For this review, use the dimensioned drawing (mm, ordinates from the lowest corner) and the shaded views. A direction names the side the tool comes from. Round coordinates to 2 decimals unless told otherwise and drop trailing zeros. Write each loop counter-clockwise with the first axis right and the second up, starting at its lowest first coordinate (ties: lowest second). Pieces come first, ordered by that corner, then holes. Notation, with made-up numbers: M 39.25,-11.75 L 81.25,-11.75 A29 cw 81.25,18.25 Z; hole C 7,56.5 d11. An arc over 180 degrees is marked long. One line per question, with ' | ' between items.
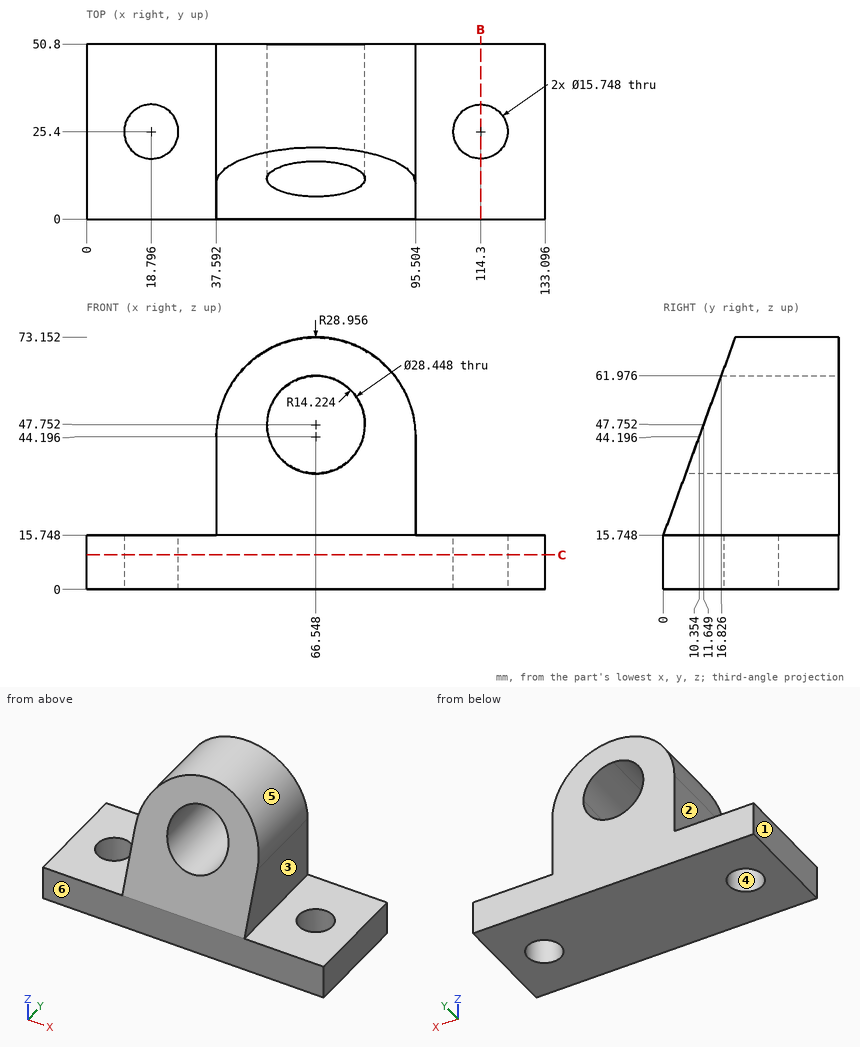
Item 1: Take a section at B-B (x = 114.3). Write out the cut boundary in (y, z) (1 decimal).
Results:
outline: M 0,0 L 17.5,0 L 17.5,15.7 L 0,15.7 Z; M 33.3,0 L 50.8,0 L 50.8,15.7 L 33.3,15.7 Z
Item 2: Machinability: for the marked faces 1, 2 and 3, which of the approach directions +Z, -Z, +X, -X, +Y, -Y give a long, thin tool a straight path to every point of the face, cutting with its end or side? Answer none if there is none.
Results:
face 1: +Z, -Z, -X, +Y, -Y | face 2: +Z, -X, +Y, -Y | face 3: +Z, +X, +Y, -Y
Item 3: Mouldability with a two-part tool opening along X and no side actions: class the marked faces 4, 5 and 6 as +X half, -X half, draft (parallel to the pull), parting line (faces both ways), or undercut.
Results:
face 4: undercut | face 5: parting line | face 6: draft
Item 4: Take a section at C-C (z = 10). Write out the cut boundary in (x, y) (1 decimal), then the cut area to 3 significant figures.
Results:
outline: M 0,0 L 133.1,0 L 133.1,50.8 L 0,50.8 Z; hole C 18.8,25.4 d15.7; hole C 114.3,25.4 d15.7 | area: 6,370 mm2
Item 5: To check wall thickness, follow line 1 along X through (y, z) = (25, 5) (1 decimal); line 2 along Z through (x, y) = (22, 48.5); line 3 along X through (y, z) = (16.5, 30.5) (1 decimal). State the ranges of each line that lie inside material, in increasing order. Write a range as from..to.
Results:
line 1: 0..10.9, 26.7..106.4, 122.2..133.1 | line 2: 0..15.75 | line 3: 37.6..95.5
Item 6: Insertion check: pin 1 Ø12.5 at (x, y) = (18.796, 25.4) entering from -Z; pin 2 Ø19 at (x, y) = (19, 25) entering from +Z; pin 3 Ø2 at (y, z) = (15.5, 60) entering from -X; pin 4 Ø23 at (y, z) = (35.5, 37) entering from -X. Each pin has a flat end and moves straight along its axis. Give the tip position at first contact, or say it passes through.
Results:
pin 1: through | pin 2: z = 15.75 | pin 3: x = 41.68 | pin 4: x = 37.59
